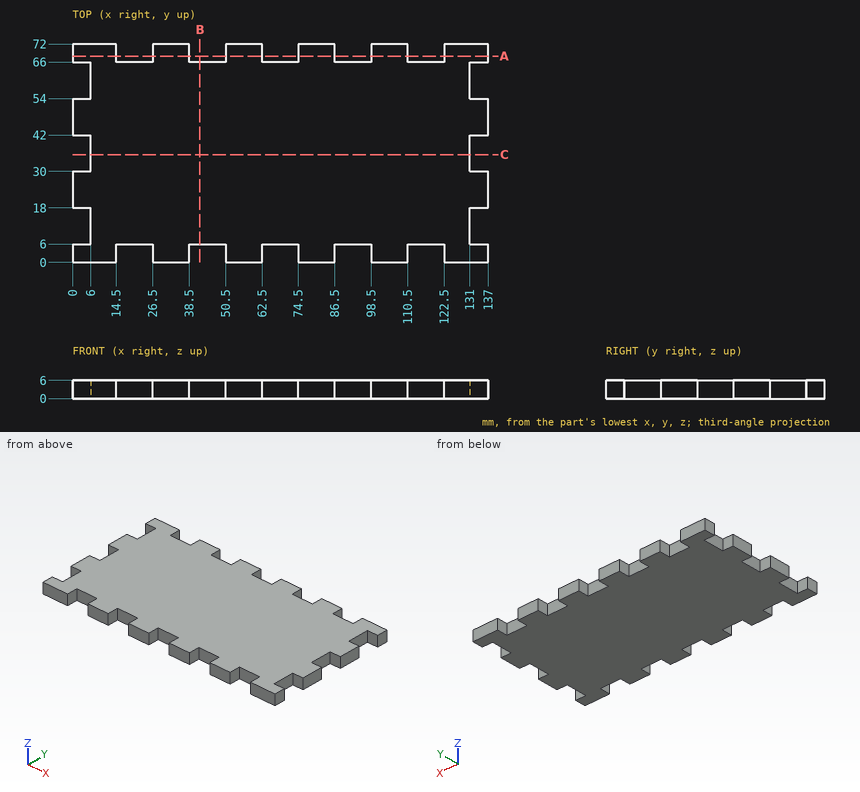
Job drawing, mm, ordinate dimensions from the low corner. One solid piece. Give positions to 0.01 mm unless a question says otherwise; leave off trailing zeros. Loops run counter-clockwise (first coordinate to the right, second up) from the corner with the lowest first, then second, coordinate; pieces in that order, holes last.
Item 1: Slice it at A-A, the plane y = 68. List the corners of the cut face in (x, z).
Answers follow:
outline: (0, 0) - (14.5, 0) - (14.5, 6) - (0, 6) - close; (26.5, 0) - (38.5, 0) - (38.5, 6) - (26.5, 6) - close; (50.5, 0) - (62.5, 0) - (62.5, 6) - (50.5, 6) - close; (74.5, 0) - (86.5, 0) - (86.5, 6) - (74.5, 6) - close; (98.5, 0) - (110.5, 0) - (110.5, 6) - (98.5, 6) - close; (122.5, 0) - (137, 0) - (137, 6) - (122.5, 6) - close
Item 2: Flat gauge pins, fed straight in: pin 1 (3 mm diameter, centred on x = 2, z = 4.5, fed in from -Y); pin 2 (1.8 mm diameter, centred on x = 116.5, z = 2.5, fed in from -Y). Where does each tip first touch, or does it go through?
Answers follow:
pin 1: stops at y = 0
pin 2: stops at y = 6
Item 3: Slice it at B-B, the plane x = 42. List the corners of the cut face in (y, z).
Answers follow:
outline: (6, 0) - (66, 0) - (66, 6) - (6, 6) - close
Item 4: Drill centre lines: line 1 (X direction, y = 4, z = 2.65); line 2 (Y direction, x = 119, z = 5.05); line 3 (X direction, y = 11.5, z = 5.55). Where is each one in solid material? Low to high.
Answers follow:
line 1: x = 0 to 14.5, 26.5 to 38.5, 50.5 to 62.5, 74.5 to 86.5, 98.5 to 110.5, 122.5 to 137
line 2: y = 6 to 66
line 3: x = 6 to 131
Item 5: Slice it at C-C, the plane y = 35.5. List the corners of the cut face in (x, z).
Answers follow:
outline: (6, 0) - (131, 0) - (131, 6) - (6, 6) - close
